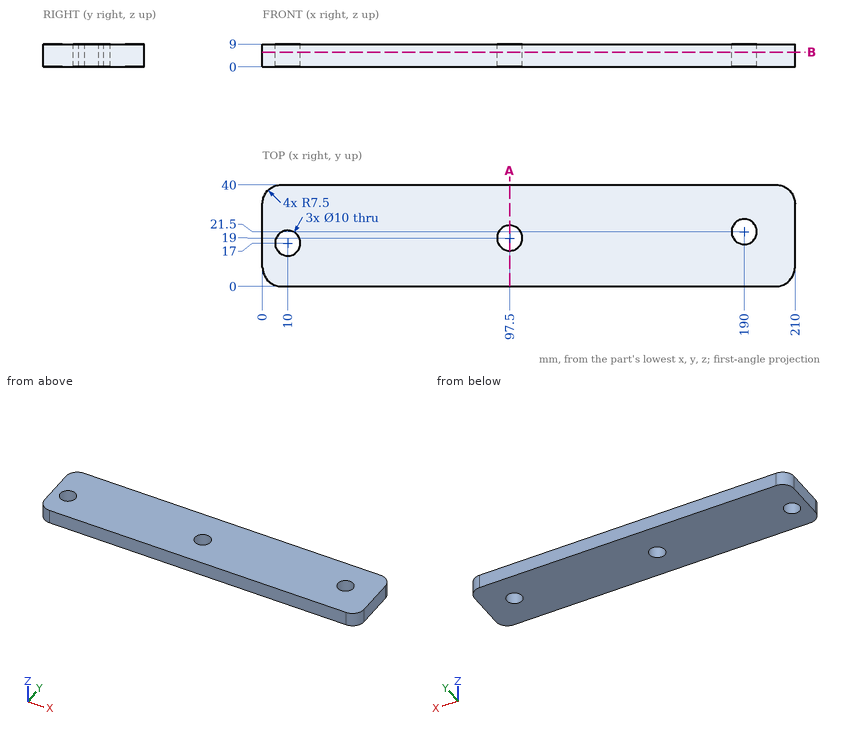
Answer from the drawing. Dimensions are ordinates in mm from the lowest x, y and z of the part. Give positions to 0.01 mm unless a question says otherwise; leave off trailing zeros. Loops run counter-clockwise (first coordinate to the right, second up) from the corner with the lowest first, then second, coordinate; pieces in that order, holes last. Notation, with made-up numbers: M -38,2.25 L 9,2.25 A24 cw 9,19.25 Z; hole C 69.5,73.25 d8. An arc over 180 degrees is marked long. One line per item, written item: value.
Q1. Find the intervals of material crossed by line 1 (X direction, y = 17, z = 5.75); line 2 (X direction, y = 15.5, z = 6.75); line 3 (X direction, y = 21.5, z = 4.25), in increasing order. Write a range as from..to.
Working result:
line 1: x = 0..5, 15..92.92, 102.08..187.82, 192.18..210
line 2: x = 0..5.23, 14.77..93.93, 101.07..210
line 3: x = 0..7.82, 12.18..93.17, 101.83..185, 195..210
Q2. A cutting plane is placed at B-B on z = 5.75. Determine the outline of the cut face in (x, y), then the cut area to 3 significant figures.
Working result:
outline: M 0,7.5 A7.5 ccw 7.5,0 L 202.5,0 A7.5 ccw 210,7.5 L 210,32.5 A7.5 ccw 202.5,40 L 7.5,40 A7.5 ccw 0,32.5 Z; hole C 10,17 d10; hole C 97.5,19 d10; hole C 190,21.5 d10
area: 8,120 mm^2
Q3. A cutting plane is placed at A-A on x = 97.5. Determine the outline of the cut face in (y, z).
Working result:
outline: M 0,0 L 14,0 L 14,9 L 0,9 Z; M 24,0 L 40,0 L 40,9 L 24,9 Z
